Verification items for this drawing (mm, ordinates from the low corner). Coordinates: 2 decimals unless noted, no trailing zeros. Loops run counter-clockwise (first coordinate to the right, second up) from the corner with the lowest first, then second, coordinate; pieces in that order, holes last. Notation, with made-up numbers: (-2.75, 85) - (28.25, 85) arc R15 ccw to (28.25, 102) - close; hole circle Ø9 at (45.5, 60.25). An arc over 180 degrees is marked (long way). One line per item, written item: value. Start each with the question number.
(1) Thickness scan on probe 1 along Z at (x, y) = (3, 2.75); probe 2 along Z at (x, y) = (2.35, 6.5) (1 decimal); probe 3 along X at (y, z) = (4, 3.2). Record the ranges inside material, lowest first. Write a range as [from, to].
(2) Section check A-A (z = 3). Record the boundary of the cut face in (x, y).
(3) Gauge pin test, flat ends, axial feed: P1, Ø3, axis at x = 3, z = 3, coming from the +Y side; P2, Ø3, axis at x = 1.5, z = 1.5, coming from the -Y side. Record the tip position at first contact, or that the pin passes through.
(4) Section check B-B (y = 8). Record the boundary of the cut face in (x, z).
(5) Draft check along Z on the marked faces 1, 2 and 3. Enter one of: +Z half, -Z half, draft (parallel to the pull), parting line (faces both ways), or undercut.
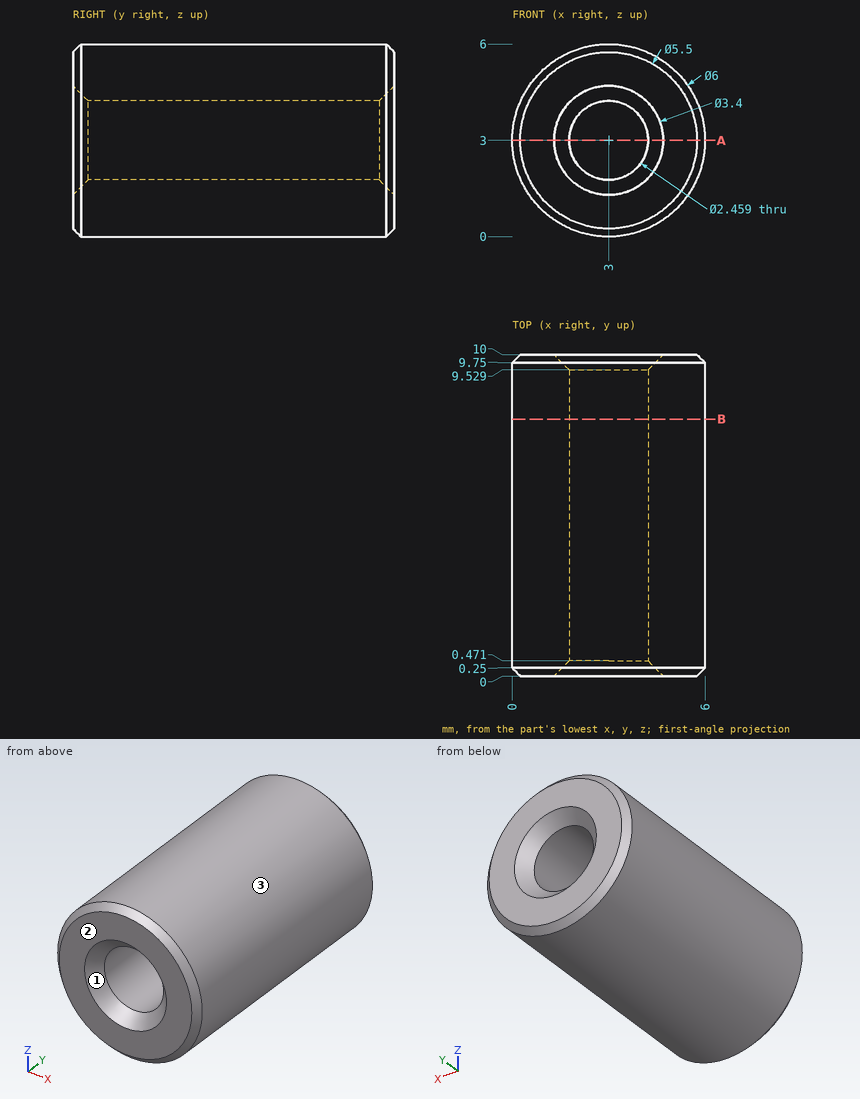
Responses:
1. probe 1: z = [0, 1.77], [4.23, 6]
1. probe 2: z = [0.1, 2], [4, 5.9]
1. probe 3: x = [0.01, 1.79], [4.21, 5.99]
2. outline: (0, 0.25) - (0.25, 0) - (1.3, 0) - (1.77, 0.47) - (1.77, 9.53) - (1.3, 10) - (0.25, 10) - (0, 9.75) - close; (4.23, 0.47) - (4.7, 0) - (5.75, 0) - (6, 0.25) - (6, 9.75) - (5.75, 10) - (4.7, 10) - (4.23, 9.53) - close
3. P1: stops at y = 9.8
3. P2: stops at y = 0
4. outline: circle Ø6 at (3, 3); hole circle Ø2.46 at (3, 3)
5. face 1: undercut
5. face 2: draft
5. face 3: parting line
